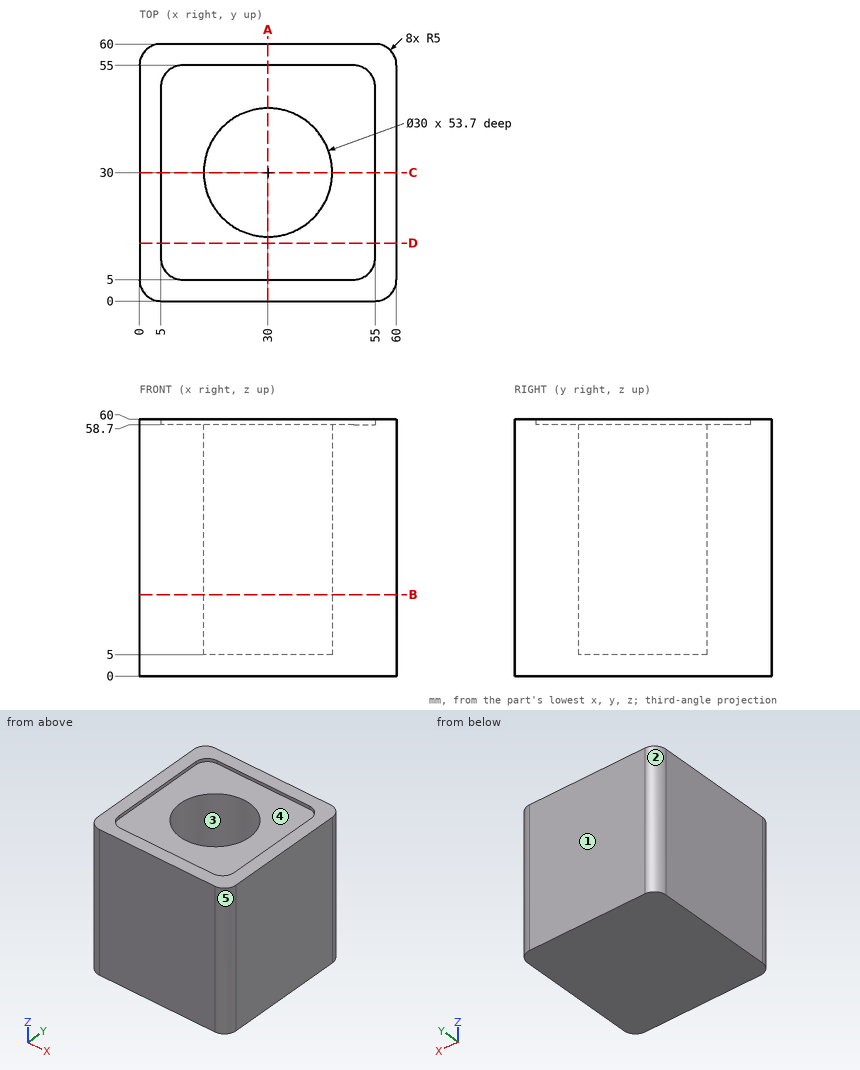
Input: dimensioned drawing with shaded views. Units: mm. Origin: part minimum x, y, z. A direction names the side the tool comes from. Round coordinates to 2 decimals unless told otherwise and drop trailing zeros. Loops run counter-clockwise (first coordinate to the right, second up) from the corner with the lowest first, then second, coordinate; pieces in that order, holes last. Notation, with made-up numbers: M 83.25,45.25 L 108.25,45.25 A5 cw 108.25,53.25 Z; hole C -15.5,49.5 d2. An arc over 180 degrees is marked long. Return JSON: item names as keys, results as strings. Group by question number.
1. Section query D-D on y = 13.5. Output: boundary loops of the cut face in (x, z).
2. Reachability of the marked faces 4 and 5 from +Z, -Z, +X, -X, +Y, -Y: full face, straight path, thin tool, end or side. Return the list, or none.
3. Section query B-B on z = 19. Output: boundary loops of the cut face in (x, y), and give its area (3 significant figures).
4. Section query A-A on x = 30. Output: boundary loops of the cut face in (y, z), and give its area (3 significant figures).
5. Pin query (flat end, axial travel): pin 1 (24 mm diameter, centred on x = 27.5, y = 34, fed in from +Z). Return the tip coordinate at first contact, or that it passes through.
6. Mould query, pull axis X, two halves, no side actions, for the marked faces 1, 2 and 3. Classes: released by +X, released by -X, zero draft, split by the parting line, or undercut.
7. Material intervals for line 1 along Y through (x, z) = (30, 21); line 2 along Z through (x, y) = (53, 39); line 3 along Y through (x, z) = (21, 11.5), sorted ascending. Write a range as from..to.
Checks:
{
 "1": {"outline": "M 0,0 L 60,0 L 60,60 L 55,60 L 55,58.7 L 5,58.7 L 5,60 L 0,60 Z"},
 "2": {"face 4": "+Z", "face 5": "+Z, -Z, +X, -Y"},
 "3": {"outline": "M 0,5 A5 ccw 5,0 L 55,0 A5 ccw 60,5 L 60,55 A5 ccw 55,60 L 5,60 A5 ccw 0,55 Z; hole C 30,30 d30", "area": "2,870 mm²"},
 "4": {"outline": "M 0,0 L 60,0 L 60,60 L 55,60 L 55,58.7 L 45,58.7 L 45,5 L 15,5 L 15,58.7 L 5,58.7 L 5,60 L 0,60 Z", "area": "1,920 mm²"},
 "5": {"pin 1": "stops at z = 58.7"},
 "6": {"face 1": "zero draft", "face 2": "released by -X", "face 3": "undercut"},
 "7": {"line 1": "y = 0..15, 45..60", "line 2": "z = 0..58.7", "line 3": "y = 0..18, 42..60"}
}
